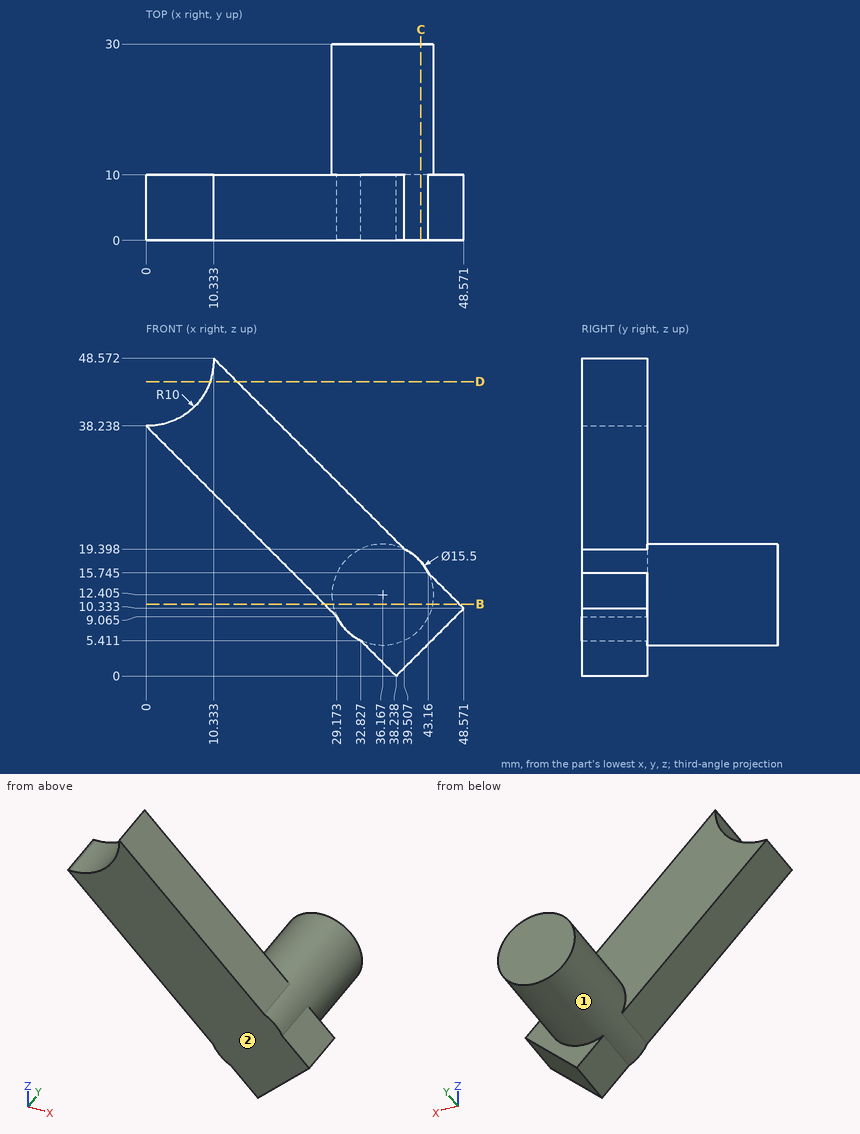
The drawing under review shows one solid part. Ordinate dimensions are in mm from its lowest x, y, z. A direction names the side the tool comes from. Give positions to 0.01 mm unless a question says otherwise; leave off trailing zeros. Order: outer loops, then holes, each group sorted by start corner. A loop starts at its lowest first (then second) coordinate and runs counter-clockwise, first axis right, second up. Notation, with made-up numbers: M 74,62.5 L 82,62.5 A27 ccw 82,100.5 Z; hole C 24,48 d8. An arc over 180 degrees is marked long. One line per question, with ' | ' between items. Start each with the question number.
Q1. Machinability: for the marked faces 1 and 2, which of the approach directions +Z, -Z, +X, -X, +Y, -Y give a long, thin tool a straight path to every point of the face, cutting with its end or side? Answer none if there is none.
Q2. We need section C-C (x = 42). Write out the cut boundary in (y, z).
Q3. We need section B-B (z = 11). Write out the cut boundary in (x, y) (1 decimal).
Q4. We need section D-D (z = 45). Write out the cut boundary in (x, y) (1 decimal), plus the area to 3 significant figures.
Q5. For L1, parallel to Z at x = 36.5, y = 16.25; L2, parallel to Y at x = 22, z = 28; L3, parallel to X at y = 4.5, z = 20 (1 decimal), list the stretches that pass through material, from the lowest coordinate up. Write a range as [from, to].
Q6. For pin 1 Ø8 at (x, z) = (33.5, 5) entering from -Y; pin 2 Ø12 at (x, y) = (19.5, 5.5) entering from -Z; pin 3 Ø4 at (x, y) = (19, 9) entering from +Z (1 decimal); pin 4 Ø2 at (x, z) = (21.5, 15.5) entering from +Y, all flat-tipped, find the tip position at first contact; note any pin that passes through.
Returned:
1) face 1: +Y | face 2: +Z, -Z, +X, -X, -Y
2) outline: M 0,3.76 L 10,3.76 L 10,7.3 L 30,7.3 L 30,17.51 L 0,17.51 Z
3) outline: M 27.2,0 L 47.9,0 L 47.9,10 L 43.8,10 L 43.8,30 L 28.5,30 L 28.5,10 L 27.2,10 Z
4) outline: M 9.8,0 L 13.9,0 L 13.9,10 L 9.8,10 Z | area: 41.1 mm2
5) L1: [4.66, 20.15] | L2: [0, 10] | L3: [18.2, 38.9]
6) pin 1: y = 0 | pin 2: z = 12.74 | pin 3: z = 41.9 | pin 4: y = 10
